Source: CAD feature listing. Evaluate the final solid. Frame: model axes, mm. A direction names the side the tool comes from. Give positions to 0.01 mm unless a question says otherwise; leave off trailing zeros. Loops run counter-clockwise (first coordinate to the right, second up) from the corner with the lowest first, then second, coordinate; pieces in that order, holes last.
Autodesk Inventor part; units mm, degrees
ref_plane "YZ Plane" through (0, 0, 0) normal (1, 0, 0) x (0, 1, 0)
ref_plane "XZ Plane" through (0, 0, 0) normal (0, 1, 0) x (-1, 0, 0)
ref_plane "XY Plane" through (0, 0, 0) normal (0, 0, 1) x (1, 0, 0)
sketch "Эскиз9" plane through (0, 0, 0) normal (0, 1, 0) x (-1, 0, 0)
  line L0 (-7.875, 10) -> (7.875, 10)
  line L1 (7.875, 10) -> (7.875, -10)
  line L2 (7.875, -10) -> (-7.875, -10)
  line L3 (-7.875, -10) -> (-7.875, 10)
  line L4 (-7.875, 10) -> (7.875, -10) construction
  line L5 (7.875, 10) -> (-7.875, -10) construction
  circle A0 centre (0.875, 4) radius 1.6
  point P0 (0, 0)
  point P1 (7.875, 0)
  dimension "d56" = 15.75
  dimension "d57" = 20
  dimension "d58" = 3.2
  dimension "d86" = 6
  dimension "d87" = 7
extrude "Выдавливание9" add sketch "Эскиз9" along normal blind 4
sketch "Эскиз10" plane through (0, 4, 0) normal (0, 1, 0) x (1, 0, 0)
  line L0 (7.875, 22) -> (-29.825, 22)
  line L1 (-29.825, 22) -> (-29.825, 10)
  line L2 (-29.825, 10) -> (7.875, 10)
  line L3 (7.875, 10) -> (7.875, 22)
  line L4 (7.875, 22) -> (-29.825, 10) construction
  line L5 (-29.825, 22) -> (7.875, 10) construction
  line L6 (7.875, 10) -> (-7.875, 10)
  line L7 (-7.875, 10) -> (-7.875, -10)
  line L8 (7.875, -10) -> (7.875, 10)
  point P0 (0, 0)
  point P1 (-10.975, 16)
  point P2 (0, 10)
  point P3 (7.875, 16)
  dimension "d71" = 37.7
  dimension "d72" = 12
extrude "Выдавливание10" add sketch "Эскиз10" against normal blind 4
sketch "Эскиз11" plane through (0, 4, 0) normal (0, 1, 0) x (1, 0, 0)
  circle A0 centre (-14.5, 13) radius 1.6 construction
  circle A1 centre (7.7, 11) radius 1.6 construction
  circle A2 centre (-27.225, 16) radius 1.6
  line L0 (-29.825, 22) -> (-29.825, 10)
  line L1 (-29.825, 10) -> (-7.875, 10)
  circle A3 centre (-5.025, 14) radius 1.6
  line L2 (7.875, -10) -> (7.875, 22)
  point P0 (-29.825, 16)
  dimension "d75" = 3.2
  dimension "d76" = 2.6
  dimension "d77" = 6
  dimension "d78" = 3.2
  dimension "d79" = 4
  dimension "d80" = 12.9
extrude "Выдавливание11" cut sketch "Эскиз11" against normal blind 4
sketch "Эскиз12" plane through (0, 4, 0) normal (0, 1, 0) x (1, 0, 0)
  line L0 (-5.875, 1) -> (-5.875, -9) construction
  line L1 (-6.875, 0) -> (-6.875, -8)
  line L2 (-4.875, -8) -> (-4.875, 0)
  arc A0 (-4.875, 0) -> (-6.875, 0) centre (-5.875, 0) ccw
  arc A1 (-6.875, -8) -> (-4.875, -8) centre (-5.875, -8) ccw
  circle A2 centre (-0.875, -4) radius 1.6
  line L3 (-0.875, -4) -> (-14.063, -4) construction
  point P0 (0, 0)
  point P1 (-5.875, -4)
  dimension "d81" = 10
  dimension "d82" = 2
  dimension "d83" = 5
extrude "Выдавливание12" cut sketch "Эскиз12" against normal blind 4
properties part number "креп_опт" material "Полипропилен"
1) Contact query for flat-ended pins moving along their axis: P1, Ø8, axis at x = -8, z = -13.5, coming from the -Y side; P2, Ø2, axis at y = 2, z = 1, coming from the -X side (3 decimals); P3, Ø3, axis at x = -5.025, z = -14, coming from the -Y side. Output: stop coordinate, or through.
Checks:
P1: stops at y = 0
P2: stops at x = -7.875
P3: passes through
2) Reachability of faces 1 (the flat face through (-11, 2, -22)), 2 (the cylindrical face through (-5.9, 2, -1)), 3 (the flat face through (-19, 2, -10)) from +Z, -Z, +X, -X, +Y, -Y: full face, straight path, thin tool, end or side. Return the list, or none.
Checks:
face 1: -Z, +X, -X, +Y, -Y
face 2: +Y, -Y
face 3: +Z, -X, +Y, -Y
3) Cut plane D-D (x = -20.5). Return loops of the section in (y, z), and give its area (3 significant figures).
Checks:
outline: (0, -22) - (4, -22) - (4, -10) - (0, -10) - close
area: 48.0 mm2
4) Cut plane A-A (z = -14). Return loops of the section in (x, y) (3 decimals), and give its area (3 significant figures).
Checks:
outline: (-29.825, 0) - (-6.625, 0) - (-6.625, 4) - (-29.825, 4) - close; (-3.425, 0) - (7.875, 0) - (7.875, 4) - (-3.425, 4) - close
area: 138 mm2
5) Cut plane C-C (z = 4). Return loops of the section in (x, y) (3 decimals), and give its area (3 significant figures).
Checks:
outline: (-7.875, 0) - (-6.875, 0) - (-6.875, 4) - (-7.875, 4) - close; (-4.875, 0) - (-2.475, 0) - (-2.475, 4) - (-4.875, 4) - close; (0.725, 0) - (7.875, 0) - (7.875, 4) - (0.725, 4) - close
area: 42.2 mm2
6) Pull-direction query (X, two-part tool) for faces 4 (the flat face through (0, 2, 10)), 5 (the flat face through (-7.875, 2, 0)), 6 (the flat face through (-4.875, 2, 4)); classes: released by +X, released by -X, zero draft, split by the parting line, or undercut.
Checks:
face 4: zero draft
face 5: released by -X
face 6: undercut
7) Ray query, probe 1 along X at (y, z) = (3, 4) (3 decimals); probe 2 along X at (y, z) = (2.9, 5) (3 decimals); probe 3 along X at (y, z) = (3.2, -14) (3 decimals). Return the intervals inside material, ascending.
Checks:
probe 1: x = -7.875 to -6.875, -4.875 to -2.475, 0.725 to 7.875
probe 2: x = -7.875 to -6.875, -4.875 to -2.124, 0.374 to 7.875
probe 3: x = -29.825 to -6.625, -3.425 to 7.875
8) Cut plane B-B (y = 1.65). Return loops of the section in (x, z) (3 decimals).
Checks:
outline: (-29.825, -22) - (7.875, -22) - (7.875, 10) - (-7.875, 10) - (-7.875, -10) - (-29.825, -10) - close; hole circle Ø3.2 at (-27.225, -16); hole (-6.875, 0) arc R1 ccw to (-4.875, 0) - (-4.875, 8) arc R1 ccw to (-6.875, 8) - close; hole circle Ø3.2 at (-5.025, -14); hole circle Ø3.2 at (-0.875, 4)
